Input: part model. Units: mm. Frame: model coordinates. Face numbers are marked on the shaded views. A direction names the side the tool comes from. Round coordinates to 2 decimals unless told otherwise and drop trailing zeros. Loops run counter-clockwise (first coordinate to the right, second up) from the corner with the lowest first, then second, coordinate; pieces in that order, holes last.
1) Section A-A, the plane x = 25. Return loops of the section in (y, z), and give its area (3 significant figures).
2) First-contact query: pin 1 (6.5 mm diameter, centred on x = 25, y = -90, fed in from +Z); pin 2 (3 mm diameter, centred on x = -39, y = 33.5, fed in from -Z); pin 3 (11 mm diameter, centred on x = -72, z = -137, fed in from +Y); pin 4 (3.5 mm diameter, centred on x = -25, y = 60, fed in from +Z). Flat tips, straight axial feed; report the tip coordinate or a pass-through.
3) Draft query along Z for the marked faces 4, 5 and 6. Return one class per face: pulls with the +Z half, pulls with the -Z half, needs draft (parallel to the pull), parting line crosses it, or undercut.
4) Section D-D, the plane x = -33. Return loops of the section in (y, z), and give its area (3 significant figures).
5) Section B-B, the plane y = -77. Return loops of the section in (x, z), and give its area (3 significant figures).
6) Section C-C, the plane x = -12.5. Return loops of the section in (y, z), and give its area (3 significant figures).
7) Access query for the marked faces 1, 2 and 3. Directions: +Z, -Z, +X, -X, +Y, -Y. A direction counts if a zero-diameter tool reaches every point of the face in a straight line with its end or side. Return the directions, or none.
8) Ray query, line 1 along X through (y, z) = (60, -41); line 2 along X through (y, z) = (35, -103.5); line 3 along Y through (x, z) = (50, -127). Return the intervals inside material, ascending.
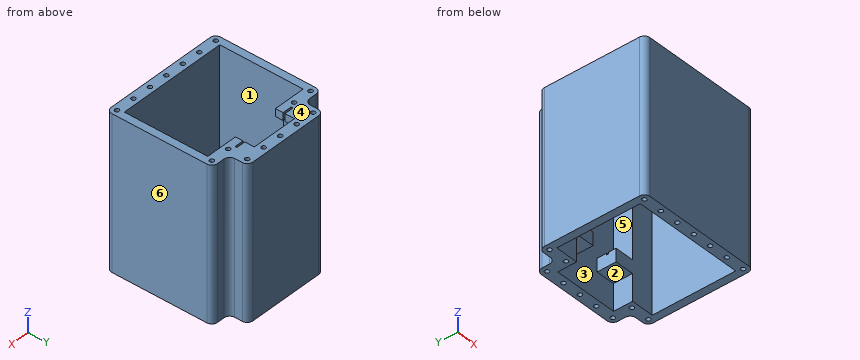
from build123d import *

# Parameters (mm, degrees)
BOSS_EXTRUDE1_DEPTH     = 200
CUT_EXTRUDE1_DEPTH      = 238.302549502
CUT_EXTRUDE1_DEPTH_BACK = 238.302549502
SKETCH2_R               = 2.8
SKETCH3_W               = 25
SKETCH3_H               = 200
BOSS_EXTRUDE2_DEPTH     = 25
SKETCH4_W               = 200
SKETCH4_H               = 2.5
CUT_EXTRUDE2_DEPTH      = 25
SKETCH5_W               = 200
SKETCH5_H               = 2.5
CUT_EXTRUDE3_DEPTH      = 25
CUT_EXTRUDE5_REACH      = 265.261
CUT_EXTRUDE7_REACH      = 251.862
SKETCH10_W              = 85
SKETCH10_H              = 35
SKETCH11_W              = 25
SKETCH11_H              = 15
BOSS_EXTRUDE3_DEPTH     = 25
CUT_EXTRUDE8_REACH      = 251.862
SKETCH12_W              = 85
SKETCH12_H              = 7.75


with BuildPart() as part:
    # Sketch1 → Boss-Extrude1 (new body)
    with BuildSketch(Plane.XY):
        with BuildLine():
            Line((-57.5, 60), (-57.5, 50))
            ThreePointArc((-57.5, 50), (-59.696699141, 44.696699141), (-65, 42.5))
            Line((-65, 42.5), (-75, 42.5))
            ThreePointArc((-75, 42.5), (-80.303300859, 40.303300859), (-82.5, 35))
            Line((-82.5, 35), (-82.5, -90))
            ThreePointArc((-82.5, -90), (-80.303300859, -95.303300859), (-75, -97.5))
            Line((-75, -97.5), (75, -97.5))
            ThreePointArc((75, -97.5), (80.303300859, -95.303300859), (82.5, -90))
            Line((82.5, -90), (82.5, 35))
            ThreePointArc((82.5, 35), (80.303300859, 40.303300859), (75, 42.5))
            Line((75, 42.5), (65, 42.5))
            ThreePointArc((65, 42.5), (59.696699141, 44.696699141), (57.5, 50))
            Line((57.5, 50), (57.5, 60))
            ThreePointArc((57.5, 60), (55.303300859, 65.303300859), (50, 67.5))
            Line((50, 67.5), (-50, 67.5))
            ThreePointArc((-50, 67.5), (-55.303300859, 65.303300859), (-57.5, 60))
        make_face()
        Polygon((-42.5, 52.5), (-42.5, 27.5), (-72.5, 27.5), (-72.5, -82.5), (72.5, -82.5), (72.5, 27.5), (42.5, 27.5), (42.5, 52.5), align=None, mode=Mode.SUBTRACT)
    extrude(amount=-BOSS_EXTRUDE1_DEPTH)

    # Sketch2 → Cut-Extrude1 (cut, two sides: drawn at the far end of the back side and taken through both)
    with BuildSketch(Plane.XY.offset(-CUT_EXTRUDE1_DEPTH_BACK)):
        with Locations((-75, 35)):
            Circle(SKETCH2_R)
        with Locations((-50, 35)):
            Circle(SKETCH2_R)
        with Locations((-50, 60)):
            Circle(SKETCH2_R)
        with Locations((50, 60)):
            Circle(SKETCH2_R)
        with Locations((25, 60)):
            Circle(SKETCH2_R)
        with Locations((0, 60)):
            Circle(SKETCH2_R)
        with Locations((-25, 60)):
            Circle(SKETCH2_R)
        with Locations((50, 35)):
            Circle(SKETCH2_R)
        with Locations((75, 35)):
            Circle(SKETCH2_R)
        with Locations((-75, -90)):
            Circle(SKETCH2_R)
        with Locations((-50, -90)):
            Circle(SKETCH2_R)
        with Locations((-25, -90)):
            Circle(SKETCH2_R)
        with Locations((0, -90)):
            Circle(SKETCH2_R)
        with Locations((25, -90)):
            Circle(SKETCH2_R)
        with Locations((50, -90)):
            Circle(SKETCH2_R)
        with Locations((75, -90)):
            Circle(SKETCH2_R)
    extrude(amount=CUT_EXTRUDE1_DEPTH + CUT_EXTRUDE1_DEPTH_BACK, mode=Mode.SUBTRACT)

    # Sketch3 → Boss-Extrude2 (add)
    with BuildSketch(Plane.XZ.offset(-52.5)):
        with Locations((-30, -100)):
            Rectangle(SKETCH3_W, SKETCH3_H)
        with Locations((30, -100)):
            Rectangle(SKETCH3_W, SKETCH3_H)
    extrude(amount=BOSS_EXTRUDE2_DEPTH)

    # Sketch4 → Cut-Extrude2 (cut)
    with BuildSketch(Plane(origin=(-17.5, 0, 0), x_dir=(0, 0, -1), z_dir=(1, 0, 0))):
        with Locations((100, 38.75)):
            Rectangle(SKETCH4_W, SKETCH4_H)
    extrude(amount=-CUT_EXTRUDE2_DEPTH, mode=Mode.SUBTRACT)

    # Sketch5 → Cut-Extrude3 (cut)
    with BuildSketch(Plane.ZY.offset(-17.5)):
        with Locations((-100, 38.75)):
            Rectangle(SKETCH5_W, SKETCH5_H)
    extrude(amount=-CUT_EXTRUDE3_DEPTH, mode=Mode.SUBTRACT)

    # Cut-Extrude5: up to this face of the body (flat: up to its plane)
    cut_extrude5_end = Plane(part.part.faces().sort_by_distance((-45, 27.5, -100))[0])
    # Sketch6 → Cut-Extrude5 (cut, up to the picked face)
    with BuildSketch(Plane.XZ.offset(-52.5), mode=Mode.PRIVATE) as cut_extrude5_sk1:
        Polygon((-30.5, 0), (-30.5, -10), (-42.5, -10), (-42.5, -60.8), (-42.5, -140), (-30.5, -140), (42.5, -140), (42.5, -60.8), (42.5, -10), (30.5, -10), (30.5, 0), (42.5, 0), (42.5, 1), (-42.5, 1), (-42.5, 0), align=None)
    cut_extrude5_tool1 = split(extrude(cut_extrude5_sk1.sketch, amount=CUT_EXTRUDE5_REACH, mode=Mode.PRIVATE), bisect_by=cut_extrude5_end, keep=Keep.BOTH, mode=Mode.PRIVATE)
    add(cut_extrude5_tool1.solids().sort_by(Axis((0, 52.5, -70.818008), (0, -1, 0)))[0], mode=Mode.SUBTRACT)

    # Cut-Extrude7: up to this face of the body (flat: up to its plane)
    cut_extrude7_end = Plane(part.part.faces().sort_by_distance((0, 52.5, -86.395348837))[0])
    # Sketch10 → Cut-Extrude7 (cut, up to the picked face)
    with BuildSketch(Plane.XZ.offset(-27.5), mode=Mode.PRIVATE) as cut_extrude7_sk1:
        with Locations((0, -182.5)):
            Rectangle(SKETCH10_W, SKETCH10_H)
    cut_extrude7_tool1 = split(extrude(cut_extrude7_sk1.sketch, amount=-CUT_EXTRUDE7_REACH, mode=Mode.PRIVATE), bisect_by=cut_extrude7_end, keep=Keep.BOTH, mode=Mode.PRIVATE)
    add(cut_extrude7_tool1.solids().sort_by(Axis((0, 27.5, -182.5), (0, 1, 0)))[0], mode=Mode.SUBTRACT)

    # Sketch11 → Boss-Extrude3 (add)
    with BuildSketch(Plane.XZ.offset(-27.5)):
        with Locations((-30, -157.5)):
            Rectangle(SKETCH11_W, SKETCH11_H)
        with Locations((30, -157.5)):
            Rectangle(SKETCH11_W, SKETCH11_H)
    extrude(amount=-BOSS_EXTRUDE3_DEPTH)

    # Cut-Extrude8: up to this face of the body (flat: up to its plane)
    cut_extrude8_end = Plane(part.part.faces().sort_by_distance((0, 52.5, -97.238878143))[0])
    # Sketch12 → Cut-Extrude8 (cut, up to the picked face)
    with BuildSketch(Plane.XZ.offset(-27.5), mode=Mode.PRIVATE) as cut_extrude8_sk1:
        with Locations((0, -143.875)):
            Rectangle(SKETCH12_W, SKETCH12_H)
    cut_extrude8_tool1 = split(extrude(cut_extrude8_sk1.sketch, amount=-CUT_EXTRUDE8_REACH, mode=Mode.PRIVATE), bisect_by=cut_extrude8_end, keep=Keep.BOTH, mode=Mode.PRIVATE)
    add(cut_extrude8_tool1.solids().sort_by(Axis((0, 27.5, -143.875), (0, 1, 0)))[0], mode=Mode.SUBTRACT)


solid = part.part
Final values:
1. outline: (-97.5, -200) - (-92.8, -200) - (-92.8, 0) - (-97.5, 0) - close; (-87.2, -200) - (-82.5, -200) - (-82.5, 0) - (-87.2, 0) - close; (27.5, -165) - (52.5, -165) - (52.5, -200) - (57.2, -200) - (57.2, 0) - (52.5, 0) - (52.5, -147.75) - (40, -147.75) - (40, -150) - (37.5, -150) - (37.5, -147.75) - (27.5, -147.75) - close; (62.8, -200) - (67.5, -200) - (67.5, 0) - (62.8, 0) - close
1. area: 4,190 mm2
2. pin 1: stops at z = 0
2. pin 2: stops at z = -165
2. pin 3: stops at y = 42.5
2. pin 4: passes through
3. face 4: pulls with the +Z half
3. face 5: undercut
3. face 6: needs draft
4. outline: (-97.5, -200) - (-82.5, -200) - (-82.5, 0) - (-97.5, 0) - close; (27.5, -165) - (52.5, -165) - (52.5, -200) - (67.5, -200) - (67.5, 0) - (40, 0) - (40, -10) - (52.5, -10) - (52.5, -147.75) - (40, -147.75) - (40, -150) - (37.5, -150) - (37.5, -147.75) - (27.5, -147.75) - close; (27.5, -10) - (37.5, -10) - (37.5, 0) - (27.5, 0) - close
4. area: 6,650 mm2
5. outline: (-82.5, -200) - (-72.5, -200) - (-72.5, 0) - (-82.5, 0) - close; (72.5, -200) - (82.5, -200) - (82.5, 0) - (72.5, 0) - close
5. area: 4,000 mm2
6. outline: (-97.5, -200) - (-82.5, -200) - (-82.5, 0) - (-97.5, 0) - close; (52.5, -200) - (67.5, -200) - (67.5, 0) - (52.5, 0) - close
6. area: 6,000 mm2
7. face 1: +Z, -Z
7. face 2: -Z
7. face 3: none
8. line 1: x = -57.5 to -52.8, -47.2 to -27.8, -22.2 to -2.8, 2.8 to 22.2, 27.8 to 47.2, 52.8 to 57.5
8. line 2: x = -82.5 to -77.8, -72.2 to -52.8, -47.2 to -42.5, 42.5 to 47.2, 52.8 to 72.2, 77.8 to 82.5
8. line 3: y = -97.5 to -92.8, -87.2 to -82.5, 27.5 to 32.2, 37.8 to 57.2, 62.8 to 67.5
